Check sheet for the modelled part. Datum: model origin and axes. Units: mm. A direction names the side the tool comes from. Coordinates: 2 decimals unless noted, no trailing zeros. Order: outer loops, then holes, each group sorted by start corner. A loop starts at its lowest first (then second) coordinate and runs counter-clockwise, first axis right, second up.
1. Cross-section at D-D (z = -146.5). Enter the section's corners in (x, y), then the cut area to 3 significant figures.
2. Set-up check for faces 4 (the flat face through (-5.339, 177, -79)), 5 (the flat face through (4.661, 171, -79)): record each of +Z, -Z, +X, -X, +Y, -Y from which the full face is reachable in a straight line by a thin tool's end or side.
3. Gauge pin test, flat ends, axial feed: pin 1 Ø12 at (y, z) = (183, -98.5) entering from -X; pin 2 Ø4 at (x, y) = (-2.5, 168.5) entering from +Z; pin 3 Ø5.5 at (y, z) = (176.77, -60) entering from -X. Record the tip position at first contact, or that the pin passes through.
4. Cross-section at A-A (z = -10). Enter the section's corners in (x, y).
5. Cross-section at C-C (y = 188). Enter the section's corners in (x, z), then the cut area to 3 significant figures.
6. Cross-section at B-B (x = -12). Enter the section's corners in (y, z).
7. Thickness scan on line 1 (Y direction, x = 2.5, z = -60); line 2 (Z direction, x = -4.25, y = 177); line 3 (X direction, y = 168.5, z = -90). Record the ranges inside material, lowest first.
8. Draft check along Y on faces 1 (the cylindrical face through (-0.409, 179.633, -59.099)), 2 (the flat face through (-2, 168, -160)), 3 (the flat face through (-13, 161.772, -79)). Enter one of: released by +Y, released by -Y, zero draft, split by the parting line, or undercut.
```python
from build123d import *

# Parameters (mm, degrees)
EXTRUDE_1_DEPTH     = 160
CUT_EXTRUDE_START   = -10
SKETCH_2_R          = 3
CUT_EXTRUDE_1_DEPTH = 262.00066797
LPATTERN1_COUNT     = 3
LPATTERN1_PITCH     = 50


with BuildPart() as part:
    # 草圖1 → 填料-伸長1 (new body)
    with BuildSketch(Plane.XY):
        Polygon((-5.338534676, 191.77157068), (-5.338534676, 161.77157068), (-20.338534676, 161.77157068), (-20.338534676, 151.77157068), (4.661465324, 151.77157068), (4.661465324, 191.77157068), align=None)
    extrude(amount=-EXTRUDE_1_DEPTH)

    # 草圖2 → 除料-伸長1 (cut)
    with BuildSketch(Plane(origin=(4.661465324, 0, 0), x_dir=(0, 0, -1), z_dir=(1, 0, 0)).offset(CUT_EXTRUDE_START)):
        with Locations(Location((110, 176.77157068, 0), (0, 0, 90))):
            Circle(SKETCH_2_R)
    cut_extrude_1 = extrude(amount=CUT_EXTRUDE_1_DEPTH, mode=Mode.SUBTRACT)

    # LPattern1: 除料-伸長1 ×3
    with Locations(*[(0, 0, i * LPATTERN1_PITCH) for i in range(1, LPATTERN1_COUNT)]):
        add(cut_extrude_1, mode=Mode.SUBTRACT)


solid = part.part
```
Data:
1. outline: (-20.34, 151.77) - (4.66, 151.77) - (4.66, 191.77) - (-5.34, 191.77) - (-5.34, 161.77) - (-20.34, 161.77) - close
1. area: 550 mm2
2. face 4: +Z, -Z, -X, +Y
2. face 5: +Z, -Z, +X, +Y, -Y
3. pin 1: stops at x = -5.34
3. pin 2: stops at z = 0
3. pin 3: passes through
4. outline: (-20.34, 151.77) - (4.66, 151.77) - (4.66, 173.77) - (-5.34, 173.77) - (-5.34, 161.77) - (-20.34, 161.77) - close; (-5.34, 179.77) - (4.66, 179.77) - (4.66, 191.77) - (-5.34, 191.77) - close
5. outline: (-5.34, -160) - (4.66, -160) - (4.66, 0) - (-5.34, 0) - close
5. area: 1,600 mm2
6. outline: (151.77, -160) - (161.77, -160) - (161.77, 0) - (151.77, 0) - close
7. line 1: y = 151.77 to 173.77, 179.77 to 191.77
7. line 2: z = -160 to -112.99, -107.01 to -62.99, -57.01 to -12.99, -7.01 to 0
7. line 3: x = -5.34 to 4.66
8. face 1: undercut
8. face 2: zero draft
8. face 3: released by +Y
